from build123d import *

# Parameters (mm, degrees)
SKETCH1_W           = 260.35
SKETCH1_H           = 241.046
BOSS_EXTRUDE1_DEPTH = 1.5875
CUT_EXTRUDE2_DEPTH  = 261.35
CUT_EXTRUDE3_DEPTH  = 261.35


with BuildPart() as part:
    # Sketch1 → Boss-Extrude1 (new body, symmetric)
    with BuildSketch(Plane(origin=(0, 0, 0), x_dir=(1, 0, 0), z_dir=(0, 1, 0))):
        Rectangle(SKETCH1_W, SKETCH1_H)
    extrude(amount=BOSS_EXTRUDE1_DEPTH, both=True)

    # Sketch3 → Cut-Extrude2 (cut, through all)
    with BuildSketch(Plane.ZY.offset(130.175)):
        Polygon((120.523, 1.5875), (117.316753604, -1.5875), (181.759591699, -66.664544845), (184.965838095, -63.489544845), align=None)
        Polygon((-120.523, 1.5875), (-115.936493069, -2.999006931), (-117.69089956, -4.753413422), (-122.277406491, -0.166906491), align=None)
    extrude(amount=-CUT_EXTRUDE2_DEPTH, mode=Mode.SUBTRACT)

    # Sketch4 → Cut-Extrude3 (cut, through all)
    with BuildSketch(Plane.ZY.offset(130.175)):
        Polygon((-95.828811288, 27.019066154), (-49.030213399, -19.779531735), (-139.395977622, -13.401975952), align=None)
    extrude(amount=-CUT_EXTRUDE3_DEPTH, mode=Mode.SUBTRACT)


solid = part.part
Geometry: final body of the model. Coordinates: model frame, mm. Coordinates: 2 decimals unless noted, no trailing zeros. Loops run counter-clockwise (first coordinate to the right, second up) from the corner with the lowest first, then second, coordinate; pieces in that order, holes last. Notation, with made-up numbers: (-34, 29.5) - (9, 29.5) arc R29 ccw to (9, 59.5) - close; hole circle Ø5 at (-24, 69). An arc over 180 degrees is marked (long way). Put each result on its own line as item: value. Start each with the question number.
Q1. Pin query (flat end, axial travel): pin 1 Ø1 at (x, y) = (67.5, 0) entering from +Z. Return the tip coordinate at first contact, or that it passes through.
Q2. Cut plane B-B, the plane x = 46. Return loops of the section in (y, z), and give its area (3 significant figures).
Q3. Cut plane A-A, the plane y = -0.25. Return loops of the section in (x, z) (3 decimals).
Q4. Line query: line 1 (Z direction, x = 22.5, y = -0.6); line 2 (Z direction, x = 100.5, y = 0.25). Output: solid intervals per line, ascending.
Filled sheet:
1. pin 1: z = 119.42
2. outline: (-1.59, -67.22) - (1.59, -70.4) - (1.59, 120.52) - (-1.59, 117.32) - close
2. area: 596 mm²
3. outline: (-130.175, -68.56) - (130.175, -68.56) - (130.175, 118.667) - (-130.175, 118.667) - close
4. line 1: -68.21 to 118.31
4. line 2: -69.06 to 119.17
